Part model, mm, in its own coordinate system. Face numbers are marked on the shaded views. A direction names the side the tool comes from. Round coordinates to 2 decimals unless told otherwise and drop trailing zeros. Loops run counter-clockwise (first coordinate to the right, second up) from the corner with the lowest first, then second, coordinate; pieces in that order, holes last.
1) Band-saw the part on D-D, the plane y = -16. Write the cut outline in (x, z), then the cut area to 3 significant figures.
2) 3-axis set-ups, long thin cutter, end or side, ignore diameter. For the marked faces 1, 2, 3, 4 and 5: which of +Z, -Z, +X, -X, +Y, -Y reach the whole face in a straight line?
3) Band-saw the part on C-C, the plane y = 0. Write the cut outline in (x, z), then the cut area to 3 significant figures.
4) Mould opens along X. For the marked faces 6 and 7 say: +X half, -X half, draft (parallel to the pull), parting line (faces both ways), or undercut.
5) Band-saw the part on A-A, the plane z = 6.5. Write the cut outline in (x, y).
6) Probe line 1 (Y direction, x = 25.5, z = 17); line 2 (X direction, y = 2.5, z = 52); line 3 (Z direction, x = -39, y = -19.5). List the from-to ranges inside material, lowest first.
7) Drop flat-ended pins along their axis: P1, Ø2, axis at x = 32, z = 41, coming from the -Y side; P2, Ø3, axis at x = 4, z = 39.5, coming from the -Y side; P3, Ø0.5, axis at y = -22, z = 4, coming from the +X side. Give the stop position or say it passes through.
8) Band-saw the part on B-B, the plane x = 29. Write the cut outline in (y, z).
from build123d import *

# Parameters (mm, degrees)
F0_W        = 52.3398779333
F0_H        = 42.6720008254
F1_DEPTH    = 8.382
F2_R        = 35.438248993
F3_DEPTH    = 58.166
F4_R        = 25.617866598
F5_DEPTH    = 76.454
F6_W        = 48.6727505922
F6_H        = 15.6686254777
F7_DEPTH    = 42.926
F8_T4_DEPTH = 224.6950187396
F8_S5_R     = 35.438248993
F8_T6_DEPTH = 117


# Not quite as in the source:
# - a fillet or chamfer that OpenCascade refuses, or shapes differently, is made with other operations: its cross-section is extruded or revolved along the edge and cut away or added


with BuildPart() as f1:
    # F0 (on Top) → F1 (new body)
    with BuildSketch(Plane.XY):
        with Locations((-29.17031385, -1.0001249611)):
            Rectangle(F0_W, F0_H)
    extrude(amount=F1_DEPTH)

    # F2 (on Top) → F3 (join)
    with BuildSketch(Plane.XY):
        with Locations((25.3365002573, 0)):
            Circle(F2_R)
    extrude(amount=F3_DEPTH)

    # F4 (on Top) → F5 (cut)
    with BuildSketch(Plane.XY):
        with Locations((25.3365002573, 0)):
            Circle(F4_R)
    extrude(amount=F5_DEPTH, mode=Mode.SUBTRACT)

    # F6 (on Top) → F7 (join)
    with BuildSketch(Plane.XY):
        with Locations((-24.3363752961, 0.8334375452)):
            Rectangle(F6_W, F6_H)
    extrude(amount=F7_DEPTH)

    # F8: chamfer of 40.64 on 1 edges, made by hand


with BuildPart() as f8_tool2:
    # F8_s3 → F8_t4 (new body)
    with BuildSketch(Plane.XZ.offset(-113.180946915)):
        Polygon((-8.0327505922, 42.926), (-48.6727505922, 2.286), (-48.6727505922, 42.926), align=None)
    extrude(amount=F8_T4_DEPTH)

    # F8_s5 → F8_t6 (cut, symmetric)
    with BuildSketch(Plane.XY.offset(22.6)):
        with Locations((25.3365002573, 0)):
            Circle(F8_S5_R)
    extrude(amount=F8_T6_DEPTH, both=True, mode=Mode.SUBTRACT)

    split(bisect_by=Plane.XY.offset(8.382), keep=Keep.TOP)


with BuildPart() as f1_1:
    add(f1.part)

    # F8_t1: cut F8_tool2
    add(f8_tool2.part, mode=Mode.SUBTRACT)


solid = f1_1.part
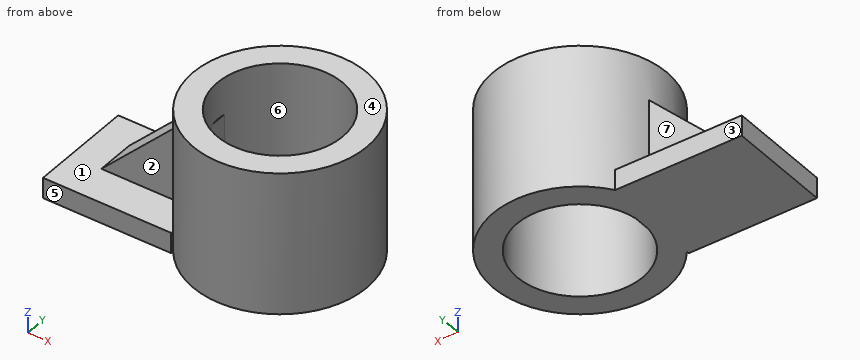
Reported:
1. outline: (-55.34, 0) - (5.33, 0) - (5.33, 58.17) - (-6.28, 58.17) - (-6.28, 8.38) - (-55.34, 8.38) - close; (45.34, 0) - (56.96, 0) - (56.96, 58.17) - (45.34, 58.17) - close
1. area: 1,760 mm2
2. face 1: +Z, -X
2. face 2: +Z, -X, -Y
2. face 3: +Z, -Z, -X, +Y
2. face 4: +Z, +X, -X, +Y, -Y
2. face 5: +Z, -Z, -X, -Y
3. outline: (-55.34, 0) - (0, 0) - (0, 42.93) - (-0.28, 42.93) - (-0.28, 58.17) - (-10.1, 58.17) - (-10.1, 40.86) - (-42.58, 8.38) - (-55.34, 8.38) - close; (50.95, 0) - (60.77, 0) - (60.77, 58.17) - (50.95, 58.17) - close
3. area: 2,060 mm2
4. face 6: undercut
4. face 7: draft
5. outline: (-55.34, -22.34) - (-3, -22.34) - (-3, -21.28) arc R35.44 ccw (long way) to (-3.69, 20.34) - (-55.34, 20.34) - close; hole (0, -3.79) arc R25.62 ccw (long way) to (0, 3.79) - close
6. line 1: y = -35.44 to -25.62, 25.62 to 35.44
6. line 2: x = -10.01 to -0.16, 50.83 to 60.69
6. line 3: z = 0 to 8.38
7. P1: stops at y = -34.98
7. P2: stops at y = -29.37
7. P3: stops at x = 53.32
8. outline: (-35.25, 0) - (-25.35, 0) - (-25.35, 58.17) - (-35.25, 58.17) - close; (25.35, 0) - (35.25, 0) - (35.25, 58.17) - (25.35, 58.17) - close
